from build123d import *

# Parameters (mm, degrees)
SKETCH_1_W      = 169
SKETCH_1_H      = 24
SKETCH_2_R      = 137.5
EXTRUDE_1_DEPTH = 27
CHAMFER_1_SIZE  = 0.5
CHAMFER_2_SIZE  = 1.999999998
CHAMFER_2_SIZE2 = 2.000000002


with BuildPart() as part:
    # 草圖1 → 旋轉1 (revolve)
    with BuildSketch(Plane.XY, mode=Mode.PRIVATE) as revolve_1_sk:
        with Locations((84.5, 44)):
            Rectangle(SKETCH_1_W, SKETCH_1_H)
    revolve(revolve_1_sk.sketch.rotate(Axis((0, 56, 0), (0, -1, 0)), 270), axis=Axis((0, 56, 0), (0, -1, 0)))

    # 草圖2 → 填料-伸長1 (add)
    with BuildSketch(Plane.XZ.offset(-32)):
        with Locations(Location((0, 0, 0), (0, 0, 270))):
            Circle(SKETCH_2_R)
    extrude(amount=EXTRUDE_1_DEPTH)

    # 草圖3 → 除料-旋轉1 (revolve, cut)
    with BuildSketch(Plane.XY, mode=Mode.PRIVATE) as cut_revolve_1_sk:
        Polygon((135, 56), (0, 56), (0, 5), (132.5, 5), (132.5, 10), (81, 10), (81, 25), (92.5, 25), (92.5, 49), (102.5, 49), (102.5, 51), (135, 51), align=None)
    revolve(cut_revolve_1_sk.sketch.rotate(Axis((0, 56, 0), (0, -1, 0)), 270), axis=Axis((0, 56, 0), (0, -1, 0)), mode=Mode.SUBTRACT)

    # 導角1
    chamfer_1_edges = [part.edges().sort_by_distance(p)[0] for p in [
        (0, 5, 137.5),
        (0, 5, 132.5),
        (0, 10, 81),
        (0, 25, 81),
        (0, 32, 169),
        (0, 56, 169),
    ]]
    chamfer(chamfer_1_edges, length=CHAMFER_1_SIZE)

    # 導角2
    chamfer_2_edges = [part.edges().sort_by_distance(p)[0] for p in [
        (0, 49, 92.5),
    ]]
    chamfer_2_side = [part.faces().sort_by_distance(p)[0] for p in [
        (0, 49, 95.399137803),
    ]]
    chamfer(chamfer_2_edges, length=CHAMFER_2_SIZE, length2=CHAMFER_2_SIZE2, reference=chamfer_2_side[0])


solid = part.part
Could you check a few things on this model? Use its own coordinates, in mm. A direction names the side the tool comes from. Give positions to 0.01 mm unless a question says otherwise; leave off trailing zeros. Loops run counter-clockwise (first coordinate to the right, second up) from the corner with the lowest first, then second, coordinate; pieces in that order, holes last. Notation, with made-up numbers: (33.25, 65.5) -> (50.25, 65.5) arc R5 ccw to (50.25, 72.5) -> close; hole circle Ø8 at (-27, 61). An arc over 180 degrees is marked (long way). Return JSON: item names as keys, results as strings.
Item 1: Which directions (+Z, -Z, +X, -X, +Y, -Y) give clear straight access to the entire face, cutting with the end or side of a thin tool? Please do faces 4 (the flat face through (112.3, 5, 71.7)), 5 (the flat face through (101, 51, -21)), 6 (the cylindrical face through (39.8, 7.78, -126.38)).
Geometry results:
{"face 4": "+Z, -Z, +X, -X, -Y", "face 5": "+Y", "face 6": "-Y"}
Item 2: If we section it at B-B on y = 17: List the corners of the cut face in (x, z) for me.
Geometry results:
{"outline": "circle Ø275 at (0, 0); hole circle Ø162 at (0, 0)"}
Item 3: If we section it at A-A on y = 37.5: List the corners of the cut face in (x, z) for me.
Geometry results:
{"outline": "circle Ø338 at (0, 0); hole circle Ø185 at (0, 0)"}
Item 4: We'd pull the mould along X, two halves only. Please class faces 1 (the flat face through (1, 32, -138)), 2 (the cylindrical face through (41.3, 18.94, -131.15)), 3 (the flat face through (61, 10, -57)): +X half, -X half, draft (parallel to the pull), parting line (faces both ways), or undercut.
Geometry results:
{"face 1": "draft", "face 2": "parting line", "face 3": "undercut"}
Item 5: I need wall thicknesses on L1, parallel to X at y = 48, z = -13; L2, parallel to X at y = 53.65, z = 0; L3, parallel to Y at x = 96, z = -134.5. Which ranges of each line are inside material? Lowest first, please. Write a range as from..to.
Geometry results:
{"L1": "x = -168.5..-92.59, 92.59..168.5", "L2": "x = -169..-135, 135..169", "L3": "y = 32..56"}
Item 6: I'm going to push flat-ended pins straight in: pin 1 (10 mm diameter, centred on x = -67.5, z = -135, fed in from -Y); pin 2 (5 mm diameter, centred on x = -17, y = 39, fed in from +Z); pin 3 (5 mm diameter, centred on x = -49, y = 49, fed in from +Z). Where does each tip first touch, or does it pass through?
Geometry results:
{"pin 1": "stops at y = 32", "pin 2": "stops at z = 168.38", "pin 3": "stops at z = 162.48"}
